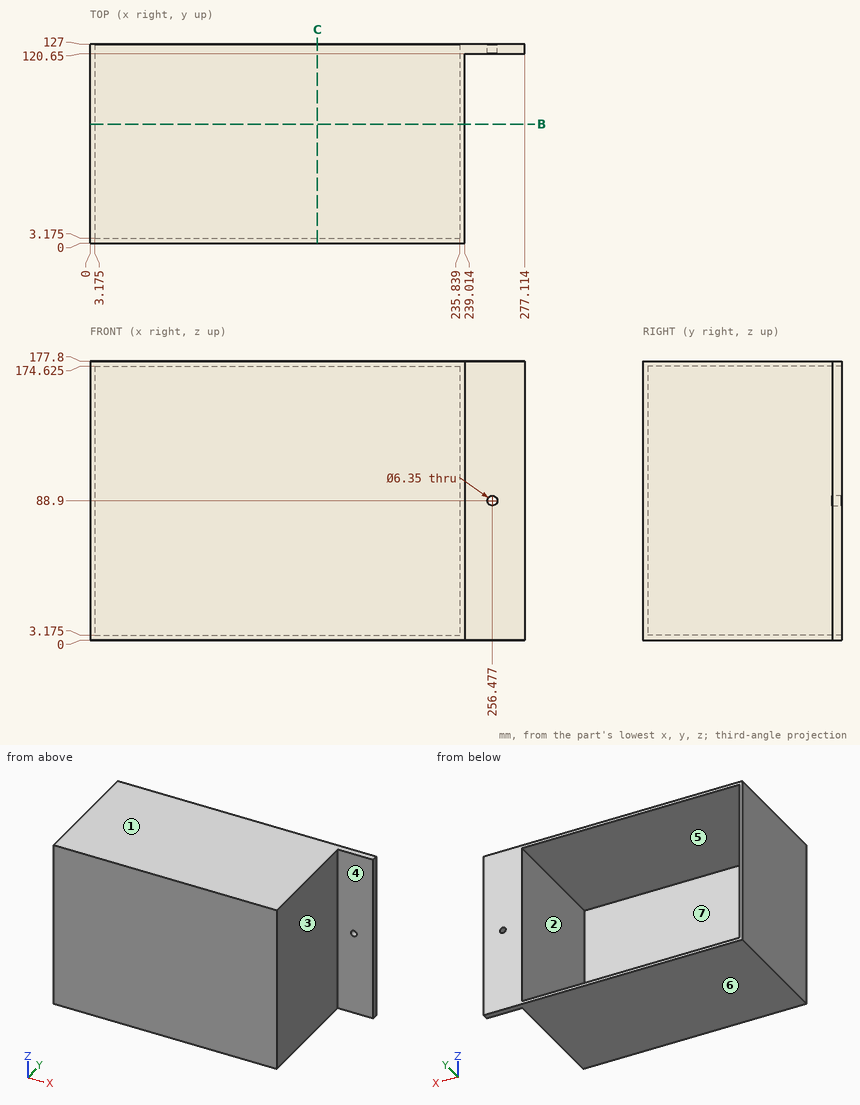
Can you work these out from the drawing? Everything is in mm from the part's minimum corner. A direction names the side the tool comes from. Round coordinates to 2 decimals unless told otherwise and drop trailing zeros. Loops run counter-clockwise (first coordinate to the right, second up) from the corner with the lowest first, then second, coordinate; pieces in that order, holes last. Notation, with made-up numbers: (-26, 40.5) - (-7, 40.5) arc R22 ccw to (-7, 62.5) - close; hole circle Ø3 at (-38.5, 9). An arc over 180 degrees is marked (long way). Answer in a Markdown table with one row per item. Add a question column.
(1) For the marked faces 1, 2 and 3, which set-ups out of +Z, -Z, +X, -X, +Y, -Y let a thin tool reach every point of the face, with its end or its side?
(2) I need wall thicknesses on line 1 along Z through (x, y) = (48, 14.5) (1 decimal); line 2 along X through (y, z) = (14, 110.5) (1 decimal); line 3 along X through (y, z) = (125, 88.9) (1 decimal). Which ranges of each line are inside material? Lowest first, please.
(3) If we section it at B-B (y = 76): Please give me the cut outline in (x, z) (1 decimal).
(4) If we mould it in two halves opening along Z, with no side actions, what happens to the marked faces 4, 5, 6 and 7? For each: pulls with the +Z half, pulls with the -Z half, needs draft (parallel to the pull), parting line crosses it, or undercut.
(5) I'm going to push flat-ended pins straight in: pin 1 (5 mm diameter, centred on y = 44.5, z = 20.5, fed in from +X); pin 2 (11.5 mm diameter, centred on x = 262.5, z = 59, fed in from -Y); pin 3 (5.5 mm diameter, centred on x = 256.48, z = 88.9, fed in from +Y); pin 4 (4 mm diameter, centred on x = 94, z = 85, fed in from +Y) (1 decimal). Where does each tip first touch, or does it pass through?
(6) If we section it at C-C (x = 145): Please give me the cut outline in (y, z) (1 decimal).
Model answer:
| question | item | result |
|---|---|---|
| 1 | face 1 | +Z, +X, -X, +Y, -Y |
| 1 | face 2 | +Y |
| 1 | face 3 | +Z, -Z, +X, -Y |
| 2 | line 1 | z = 0 to 3.2, 174.6 to 177.8 |
| 2 | line 2 | x = 0 to 3.2, 235.8 to 239 |
| 2 | line 3 | x = 0 to 3.2, 235.8 to 253.3, 259.7 to 277.1 |
| 3 | outline | (0, 0) - (239, 0) - (239, 177.8) - (0, 177.8) - close; hole (3.2, 3.2) - (235.8, 3.2) - (235.8, 174.6) - (3.2, 174.6) - close |
| 4 | face 4 | needs draft |
| 4 | face 5 | undercut |
| 4 | face 6 | pulls with the -Z half |
| 4 | face 7 | undercut |
| 5 | pin 1 | stops at x = 239.01 |
| 5 | pin 2 | stops at y = 120.65 |
| 5 | pin 3 | passes through |
| 5 | pin 4 | stops at y = 3.2 |
| 6 | outline | (0, 0) - (127, 0) - (127, 3.2) - (3.2, 3.2) - (3.2, 174.6) - (127, 174.6) - (127, 177.8) - (0, 177.8) - close |
